Work out the finished part from the listing and answer in its coordinate system (mm). A direction names the side the tool comes from. Give positions to 0.01 mm unless a question says otherwise; leave off trailing zeros. Loops run counter-clockwise (first coordinate to the right, second up) from the corner with the lowest first, then second, coordinate; pieces in that order, holes last. Notation, with made-up numbers: (-30.75, -4.5) - (-18.75, -4.5) arc R12 ccw to (-18.75, 18.5) - close; hole circle Ø6 at (5, 10). An arc over 180 degrees is marked (long way). One line per question, with ' | ' between items.
from build123d import *

# Parameters (mm, degrees)
SKETCH1_W           = 9
SKETCH1_H           = 9
SKETCH1_R           = 1.5
SKETCH1_W_2         = 16
SKETCH1_H_2         = 23
BOSS_EXTRUDE1_DEPTH = 15
SKETCH2_W           = 10
SKETCH2_H           = 10
SKETCH2_W_2         = 8.5
SKETCH2_H_2         = 2
SKETCH2_W_3         = 9
SKETCH2_H_3         = 12
CUT_EXTRUDE1_DEPTH  = 20


with BuildPart() as part:
    # Sketch1 → Boss-Extrude1 (new body)
    # profile 1 of 3: a face of its own
    with BuildSketch(Plane.XY):
        with Locations((-12.5, 0)):
            Rectangle(SKETCH1_W, SKETCH1_H)
        with Locations((-12.5, 0)):
            Circle(SKETCH1_R, mode=Mode.SUBTRACT)
    # profile 2 of 3: a face of its own
    with BuildSketch(Plane.XY):
        Rectangle(SKETCH1_W_2, SKETCH1_H_2)
    # profile 3 of 3: a face of its own
    with BuildSketch(Plane.XY):
        with Locations((12.5, 0)):
            Rectangle(SKETCH1_W, SKETCH1_H)
        with Locations((12.5, 0)):
            Circle(SKETCH1_R, mode=Mode.SUBTRACT)
    extrude(amount=BOSS_EXTRUDE1_DEPTH)

    # Sketch2 → Cut-Extrude1 (cut)
    with BuildSketch(Plane.XZ.offset(11.5)):
        with Locations((0, 7)):
            Rectangle(SKETCH2_W, SKETCH2_H)
        with Locations((0, 1)):
            Rectangle(SKETCH2_W_2, SKETCH2_H_2)
        with Locations((12.5, 9)):
            Rectangle(SKETCH2_W_3, SKETCH2_H_3)
        with Locations((-12.5, 9)):
            Rectangle(SKETCH2_W_3, SKETCH2_H_3)
    extrude(amount=-CUT_EXTRUDE1_DEPTH, mode=Mode.SUBTRACT)


solid = part.part
1. Determine the mould class of faces 6 (the flat face through (17, 0, 1)), 7 (the cylindrical face through (-14, 0, 1)), 8 (the flat face through (-17, 0, 1)) for opening direction X: +X half, -X half, draft (parallel to the pull), parting line (faces both ways), or undercut.
Evaluation:
face 6: +X half | face 7: undercut | face 8: -X half
2. Consider L1, parallel to X at y = 0, z = 1.7; L2, parallel to Y at x = -12.5, z = 2.05; L3, parallel to X at y = 0, z = 2.15. Determine where each line is inside the solid, lowest interval first.
Evaluation:
L1: -17 to -14, -11 to -4.25, 4.25 to 11, 14 to 17 | L2: -4.5 to -1.5, 1.5 to 4.5 | L3: -17 to -14, -11 to -5, 5 to 11, 14 to 17
3. Find section A-A on x = 12.5. Write down the section's boundary in (y, z).
Evaluation:
outline: (-4.5, 0) - (-1.5, 0) - (-1.5, 3) - (-4.5, 3) - close; (1.5, 0) - (4.5, 0) - (4.5, 3) - (1.5, 3) - close
4. Which of the six approach directions +Z, -Z, +X, -X, +Y, -Y give full straight-line access (tool end or side, diameter ignored) to faces 1 (the flat face through (12, 4.5, 1)), 2 (the flat face through (-14, -1, 3)), 3 (the flat face through (-4.25, -2, 1)), 4 (the flat face through (12, -4.5, 1)), 5 (the flat face through (5, -2, 7))?
Evaluation:
face 1: +Z, -Z, +X, +Y | face 2: +Z, -X, +Y, -Y | face 3: -Z, -Y | face 4: +Z, -Z, +X, -Y | face 5: -Y
5. Flat-ended cylindrical pins translate along their axes: pin 1 (3.5 mm diameter, centred on x = 12.5, y = 0, fed in from -Z); pin 2 (2.5 mm diameter, centred on x = -12.5, y = 0, fed in from -Z); pin 3 (5 mm diameter, centred on y = 2, z = 8, fed in from +X); pin 4 (1.5 mm diameter, centred on x = 11.5, z = 1.5, fed in from -Y). Find the tip coordinate at first contact, or state that the pin passes through.
Evaluation:
pin 1: z = 0 | pin 2: through | pin 3: x = 8 | pin 4: y = -4.5
6. Find section D-D on y = -8.5. Write down the section's boundary in (x, z), then the cut area to 3 significant figures.
Evaluation:
outline: (-8, 0) - (-4.25, 0) - (-4.25, 2) - (-5, 2) - (-5, 12) - (5, 12) - (5, 2) - (4.25, 2) - (4.25, 0) - (8, 0) - (8, 15) - (-8, 15) - close | area: 123 mm2
7. Find section C-C on z = 1. Write down the section's boundary in (x, y).
Evaluation:
outline: (-17, -4.5) - (-8, -4.5) - (-8, -11.5) - (-4.25, -11.5) - (-4.25, 8.5) - (4.25, 8.5) - (4.25, -11.5) - (8, -11.5) - (8, -4.5) - (17, -4.5) - (17, 4.5) - (8, 4.5) - (8, 11.5) - (-8, 11.5) - (-8, 4.5) - (-17, 4.5) - close; hole circle Ø3 at (-12.5, 0); hole circle Ø3 at (12.5, 0)
8. Find section B-B on y = 0. Write down the section's boundary in (x, z), then the cut area to 3 significant figures.
Evaluation:
outline: (-17, 0) - (-14, 0) - (-14, 3) - (-17, 3) - close; (-11, 0) - (-4.25, 0) - (-4.25, 2) - (-5, 2) - (-5, 12) - (5, 12) - (5, 2) - (4.25, 2) - (4.25, 0) - (11, 0) - (11, 3) - (8, 3) - (8, 15) - (-8, 15) - (-8, 3) - (-11, 3) - close; (14, 0) - (17, 0) - (17, 3) - (14, 3) - close | area: 159 mm2
